from build123d import *

# Parameters (mm, degrees)
SKETCH1_W               = 120
SKETCH1_H               = 50
BOSS_EXTRUDE1_DEPTH     = 20
CUT_EXTRUDE1_DEPTH      = 69.007352544
CUT_EXTRUDE1_DEPTH_BACK = 69.007352544
SKETCH2_R               = 1.25
SKETCH3_R               = 2.5
CUT_EXTRUDE2_DEPTH      = 5
CUT_EXTRUDE3_REACH      = 82.623
SKETCH4_R               = 7.5
CUT_EXTRUDE4_REACH      = 70.007
SKETCH5_R               = 2


with BuildPart() as part:
    # Sketch1 → Boss-Extrude1 (new body)
    with BuildSketch(Plane.XY):
        Rectangle(SKETCH1_W, SKETCH1_H)
    extrude(amount=BOSS_EXTRUDE1_DEPTH)

    # Sketch2 → Cut-Extrude1 (cut, two sides: drawn at the far end of the back side and taken through both)
    with BuildSketch(Plane.XY.offset(20).offset(-CUT_EXTRUDE1_DEPTH_BACK)):
        with Locations((-56.5, 10)):
            Circle(SKETCH2_R)
        with Locations((-31.5, 10)):
            Circle(SKETCH2_R)
        with Locations((-56.5, -10)):
            Circle(SKETCH2_R)
        with Locations((-31.5, -10)):
            Circle(SKETCH2_R)
        with Locations((56.5, -10)):
            Circle(SKETCH2_R)
        with Locations((31.5, -10)):
            Circle(SKETCH2_R)
        with Locations((31.5, 10)):
            Circle(SKETCH2_R)
        with Locations((56.5, 10)):
            Circle(SKETCH2_R)
    extrude(amount=CUT_EXTRUDE1_DEPTH + CUT_EXTRUDE1_DEPTH_BACK, mode=Mode.SUBTRACT)

    # Sketch3 → Cut-Extrude2 (cut)
    with BuildSketch(Plane.XY.offset(20)):
        with Locations((-56.5, 10)):
            Circle(SKETCH3_R)
        with Locations((-31.5, 10)):
            Circle(SKETCH3_R)
        with Locations(Location((-56.5, -10, 0), (0, 0, 180))):
            Circle(SKETCH3_R)
        with Locations(Location((-31.5, -10, 0), (0, 0, 180))):
            Circle(SKETCH3_R)
        with Locations(Location((56.5, 10, 0), (0, 0, 180))):
            Circle(SKETCH3_R)
        with Locations(Location((31.5, 10, 0), (0, 0, 180))):
            Circle(SKETCH3_R)
        with Locations((31.5, -10)):
            Circle(SKETCH3_R)
        with Locations((56.5, -10)):
            Circle(SKETCH3_R)
    extrude(amount=-CUT_EXTRUDE2_DEPTH, mode=Mode.SUBTRACT)

    # Sketch4 → Cut-Extrude3 (cut, up to next)
    with BuildSketch(Plane(origin=(0, 25, 0), x_dir=(1, 0, 0), z_dir=(0, 1, 0)), mode=Mode.PRIVATE) as cut_extrude3_sk1:
        with Locations(Location((0, -10, 0), (0, 0, 180))):
            Circle(SKETCH4_R)
    cut_extrude3_tool1 = extrude(cut_extrude3_sk1.sketch, amount=-CUT_EXTRUDE3_REACH, mode=Mode.PRIVATE) & part.part
    add(cut_extrude3_tool1.solids().sort_by_distance((0, 25, 10))[0], mode=Mode.SUBTRACT)

    # Sketch5 → Cut-Extrude4 (cut, up to next)
    with BuildSketch(Plane.XY.offset(20), mode=Mode.PRIVATE) as cut_extrude4_sk1:
        with Locations((42.5, 10)):
            Circle(SKETCH5_R)
    cut_extrude4_tool1 = extrude(cut_extrude4_sk1.sketch, amount=-CUT_EXTRUDE4_REACH, mode=Mode.PRIVATE) & part.part
    # Sketch5 → Cut-Extrude4 (cut, up to next)
    with BuildSketch(Plane.XY.offset(20), mode=Mode.PRIVATE) as cut_extrude4_sk2:
        with Locations((42.5, -10)):
            Circle(SKETCH5_R)
    cut_extrude4_tool2 = extrude(cut_extrude4_sk2.sketch, amount=-CUT_EXTRUDE4_REACH, mode=Mode.PRIVATE) & part.part
    # Sketch5 → Cut-Extrude4 (cut, up to next)
    with BuildSketch(Plane.XY.offset(20), mode=Mode.PRIVATE) as cut_extrude4_sk3:
        with Locations((-42.5, -10)):
            Circle(SKETCH5_R)
    cut_extrude4_tool3 = extrude(cut_extrude4_sk3.sketch, amount=-CUT_EXTRUDE4_REACH, mode=Mode.PRIVATE) & part.part
    # Sketch5 → Cut-Extrude4 (cut, up to next)
    with BuildSketch(Plane.XY.offset(20), mode=Mode.PRIVATE) as cut_extrude4_sk4:
        with Locations((-42.5, 10)):
            Circle(SKETCH5_R)
    cut_extrude4_tool4 = extrude(cut_extrude4_sk4.sketch, amount=-CUT_EXTRUDE4_REACH, mode=Mode.PRIVATE) & part.part
    add(cut_extrude4_tool1.solids().sort_by_distance((42.5, 10, 20))[0], mode=Mode.SUBTRACT)
    add(cut_extrude4_tool2.solids().sort_by_distance((42.5, -10, 20))[0], mode=Mode.SUBTRACT)
    add(cut_extrude4_tool3.solids().sort_by_distance((-42.5, -10, 20))[0], mode=Mode.SUBTRACT)
    add(cut_extrude4_tool4.solids().sort_by_distance((-42.5, 10, 20))[0], mode=Mode.SUBTRACT)


solid = part.part
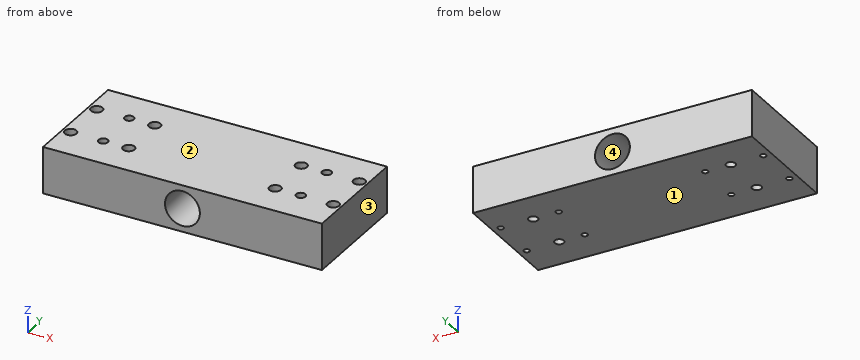
Part model, mm, in its own coordinate system. Face numbers are marked on the shaded views. Round coordinates to 2 decimals unless told otherwise and drop trailing zeros. Write each loop counter-clockwise with the first axis right and the second up, starting at its lowest first coordinate (ties: lowest second). Pieces come first, ordered by that corner, then holes. Notation, with made-up numbers: M 8,-26 L 40,-26 A30 ccw 40,11 Z; hole C -14.5,56.25 d5. An arc over 180 degrees is marked long. Return JSON: item names as keys, results as strings. Group by question number.
(1) Saw through at B-B on z = 10. Count the separate pieces of the cut face and the enclosed holes in it, then the cut area to 3 significant figures.
(2) Pin check, flat tips, straight feed: pin 1 Ø3 at (x, y) = (-31.5, 10) entering from -Z; pin 2 Ø4 at (x, y) = (31.5, -10) entering from +Z. Stop position of each tip, or through.
(3) Drill centre lines: probe 1 along Y at (x, z) = (42.5, 8); probe 2 along Y at (x, z) = (31.5, 9.5); probe 3 along X at (y, z) = (0, 10.25). Where is each one in solid material? Low to high.
(4) Saw through at C-C on x = 0. Write the cut outline in (y, z), then the cut area to 3 significant figures.
(5) Two-plate mould, pull along Z, no slides. Class the marked faces 1, 2, 3 and 4: +Z half, -Z half, draft (parallel to the pull), parting line (faces both ways), or undercut.
(6) Saw through at A-A on x = 42.5. Write the cut outline in (y, z).
Returned:
{
 "1": {"separate pieces": "2", "enclosed holes": "12", "area": "5,160 mm²"},
 "2": {"pin 1": "z = 0", "pin 2": "z = 15"},
 "3": {"probe 1": "-25 to -12, -8 to 8, 12 to 25", "probe 2": "-25 to -11.25, -8.75 to 8.75, 11.25 to 25", "probe 3": "-60 to -7.5, 7.5 to 60"},
 "4": {"outline": "M -25,0 L 25,0 L 25,2.5 L -25,2.5 Z; M -25,17.5 L 25,17.5 L 25,20 L -25,20 Z", "area": "250 mm²"},
 "5": {"face 1": "-Z half", "face 2": "+Z half", "face 3": "draft", "face 4": "undercut"},
 "6": {"outline": "M -25,0 L -12,0 L -12,20 L -25,20 Z; M -8,0 L 8,0 L 8,20 L -8,20 Z; M 12,0 L 25,0 L 25,20 L 12,20 Z"}
}
